The listing builds one solid part. Answer for the finished solid, in the listing's coordinates (mm). Round coordinates to 2 decimals unless told otherwise and drop trailing zeros. Write each loop counter-clockwise with the first axis right and the second up, starting at its lowest first coordinate (ties: lowest second). Pieces come first, ordered by that corner, then holes. Notation, with made-up numbers: M 53,20.25 L 86,20.25 A18 ccw 86,46.25 Z; hole C 73.5,19.5 d6. An arc over 180 degrees is marked long. Write each question's results on one line, items separated by ' | '.
from build123d import *

# Parameters (mm, degrees)
EXTRUSION1_DEPTH        = 328
ESQUISSE2_R             = 2.8
ENL_V_MAT_EXTRU_1_DEPTH = 329
CONG_1_R                = 0.5
CONG_2_R                = 1


with BuildPart() as part:
    # Esquisse1 → Extrusion1 (new body)
    with BuildSketch(Plane.XY):
        Polygon((-2.8, 11), (-2.8, 9.3), (-8.097918472, 9.3), (-3.297918472, 4.5), (3.297918472, 4.5), (8.097918472, 9.3), (2.8, 9.3), (2.8, 11), (11, 11), (11, 2.8), (9.3, 2.8), (9.3, 8.097918472), (4.5, 3.297918472), (4.5, -3.297918472), (9.3, -8.097918472), (9.3, -2.8), (11, -2.8), (11, -11), (2.8, -11), (2.8, -9.3), (8.097918472, -9.3), (3.297918472, -4.5), (-3.297918472, -4.5), (-8.097918472, -9.3), (-2.8, -9.3), (-2.8, -11), (-11, -11), (-11, -2.8), (-9.3, -2.8), (-9.3, -8.097918472), (-4.5, -3.297918472), (-4.5, 3.297918472), (-9.3, 8.097918472), (-9.3, 2.8), (-11, 2.8), (-11, 11), align=None)
    extrude(amount=EXTRUSION1_DEPTH)

    # Esquisse2 → Enlèv. mat.-Extru.1 (cut, through all)
    with BuildSketch(Plane(origin=(0, 0, 0), x_dir=(-1, 0, 0), z_dir=(0, 0, -1))):
        Circle(ESQUISSE2_R)
    extrude(amount=-ENL_V_MAT_EXTRU_1_DEPTH, mode=Mode.SUBTRACT)

    # Congé1
    cong_1_edges = [part.edges().sort_by_distance(p)[0] for p in [
        (-11, 11, 164),
        (11, 11, 164),
        (11, -11, 164),
        (-11, -11, 164),
    ]]
    fillet(cong_1_edges, radius=CONG_1_R)

    # Congé2
    cong_2_edges = [part.edges().sort_by_distance(p)[0] for p in [
        (-4.5, -3.297918472, 164),
        (-4.5, 3.297918472, 164),
        (-3.297918472, 4.5, 164),
        (3.297918472, 4.5, 164),
        (4.5, 3.297918472, 164),
        (4.5, -3.297918472, 164),
        (3.297918472, -4.5, 164),
        (-3.297918472, -4.5, 164),
    ]]
    fillet(cong_2_edges, radius=CONG_2_R)


solid = part.part
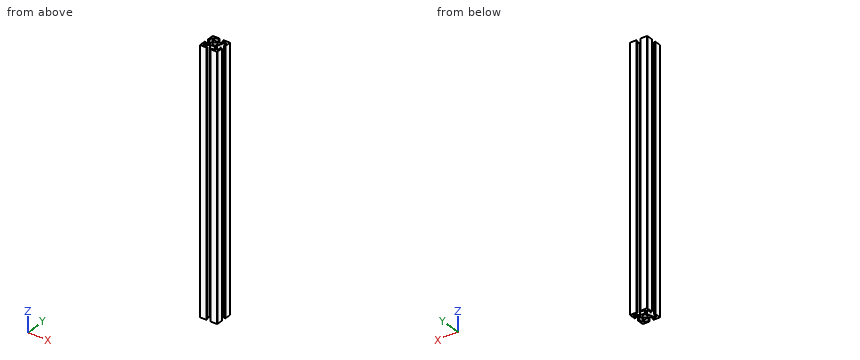
1) Each of these flat-tipped pins is pushed along its axis until it touches: pin 1 (4.5 mm diameter, centred on x = 0, z = 202.5, fed in from -Y); pin 2 (4.5 mm diameter, centred on y = -0.5, z = 104, fed in from +X). Where does it stop, or does it pass through?
Return value:
pin 1: y = -4.5 | pin 2: x = 4.5
2) Find the intervals of material crossed by line 1 (X direction, y = 9.5, z = 85.5); line 2 (Y direction, x = 0, z = 257); line 3 (Y direction, x = -7, z = 255), in increasing order.
Return value:
line 1: -11 to -2.8, 2.8 to 11 | line 2: -4.5 to -2.8, 2.8 to 4.5 | line 3: -11 to -9.3, -8.2 to -5.8, 5.8 to 8.2, 9.3 to 11
3) Section A-A (y = 0) is taken. Determine the outline of the cut face in (x, z), then the cut area to 3 significant figures.
Return value:
outline: M -4.5,0 L -2.8,0 L -2.8,328 L -4.5,328 Z; M 2.8,0 L 4.5,0 L 4.5,328 L 2.8,328 Z | area: 1,120 mm²
